Autodesk Inventor part; units mm, degrees
ref_plane "YZ Plane" through (0, 0, 0) normal (1, 0, 0) x (0, 1, 0)
ref_plane "XZ Plane" through (0, 0, 0) normal (0, 1, 0) x (-1, 0, 0)
ref_plane "XY Plane" through (0, 0, 0) normal (0, 0, 1) x (1, 0, 0)
sketch "Sketch1" plane through (0, 0, 0) normal (1, 0, 0) x (0, 1, 0)
  line L0 (-105, -75) -> (105, -75)
  line L1 (105, -75) -> (105, 75)
  line L2 (105, 75) -> (-105, 75)
  line L3 (-105, 75) -> (-105, -75)
  line L4 (-105, -75) -> (105, 75) construction
  line L5 (105, -75) -> (-105, 75) construction
  point P0 (0, 0)
  point P1 (0, 0)
  point P2 (0, 0)
  dimension "d0" = 150
  dimension "d1" = 210
extrude "Extrusion1" add sketch "Sketch1" along normal blind 6
sketch "Sketch2" plane through (6, 0, 0) normal (1, 0, 0) x (0, 0, -1)
  line L0 (75, -105) -> (75, 105)
  line L1 (-75, -105) -> (75, -105)
  line L2 (75, 105) -> (100, 105)
  line L3 (100, 105) -> (100, 80)
  line L4 (100, 80) -> (75, 30)
  line L5 (75, 30) -> (75, 105)
  line L6 (75, -105) -> (75, -5)
  line L7 (75, -5) -> (100, -55)
  line L8 (100, -55) -> (100, -105)
  line L9 (100, -105) -> (75, -105)
  point P0 (0, 0)
  dimension "d4" = 25
  dimension "d5" = 50
  dimension "d25" = 50
extrude "Extrusion2" add sketch "Sketch2" against normal blind 6
sketch "Sketch3" plane through (6, 0, 0) normal (1, 0, 0) x (0, 0, -1)
  line L0 (-75, 105) -> (-75, -105)
  line L1 (-75, -105) -> (100, -105)
  line L2 (100, -105) -> (100, -55)
  line L3 (-75, 105) -> (-25, -105)
  line L4 (-25, -105) -> (-75, -105)
  line L5 (-75, -105) -> (-75, 105)
  point P0 (0, 0)
  dimension "d8" = 50
extrude "Extrusion3" cut sketch "Sketch3" against normal through all
sketch "Sketch4" plane through (6, 0, 0) normal (1, 0, 0) x (0, 0, -1)
  line L0 (-25, -105) -> (100, -105)
  line L1 (100, -105) -> (100, -55)
  line L2 (-16.9, -105) -> (91.9, -105)
  line L3 (91.9, -105) -> (91.9, -111)
  line L4 (91.9, -111) -> (-16.9, -111)
  line L5 (-16.9, -111) -> (-16.9, -105)
  point P0 (0, 0)
  dimension "d11" = 8.1
  dimension "d12" = 8.1
  dimension "d13" = 6
extrude "Extrusion4" add sketch "Sketch4" against normal blind 6
sketch "Sketch5" plane through (6, 0, 0) normal (1, 0, 0) x (0, 0, -1)
  line L0 (-75, 105) -> (-25, -105)
  line L1 (91.9, -105) -> (100, -105)
  line L2 (100, 80) -> (100, 105)
  line L3 (100, 105) -> (-75, 105)
  circle A0 centre (-12.5, -92.5) radius 2.7
  circle A1 centre (87.5, -67.5) radius 2.7
  circle A2 centre (87.5, 92.5) radius 2.7
  circle A3 centre (-56.5476, 92.5) radius 2.7
  line L4 (-12.5, -92.5) -> (-56.5476, 92.5) construction
  line L5 (-25, -105) -> (-16.9, -105)
  point P0 (0, 0)
  dimension "d17" = 12.5
  dimension "d18" = 12.5
  dimension "d19" = 12.5
  dimension "d21" = 5.4
  dimension "d22" = 37.5
  dimension "d26" = 12.5
extrude "Extrusion5" cut sketch "Sketch5" against normal through all
fillet "Fillet1" radius 2 10 edges at (3, -111, 16.9) (3, -105, 25) (3, -111, -91.9) (3, -105, -100) (3, 105, 75) (3, 105, -100) (3, 80, -100) (3, 30, -75) (3, -5, -75) (3, -55, -100)
properties part number "BottomRightSide"
The listing builds one solid part. Answer for the finished solid, in the listing's coordinates (mm). A direction names the side the tool comes from. Coordinates: 2 decimals unless noted, no trailing zeros. Order: outer loops, then holes, each group sorted by start corner. A loop starts at its lowest first (then second) coordinate and runs counter-clockwise, first axis right, second up. Notation, with made-up numbers: (79.25, 36) -> (122.25, 36) arc R18 ccw to (122.25, 64) -> close; hole circle Ø5 at (-26.5, 70.25). An arc over 180 degrees is marked (long way). Answer in a Markdown table with one row per item. Add a question column.
Item 1: Which of the six approach directions +Z, -Z, +X, -X, +Y, -Y give full straight-line access (tool end or side, diameter ignored) to faces 1 (the face through (3.042, -95.136, 13.085)), 2 (the face through (3, -105, -95)), 3 (the face through (3, -105, 20)), 4 (the face through (3, 92, -100)), 5 (the face through (3.04, -29.66, -87.33))?
Item 2: Find section C-C (z = -87.5). Write down the section's boundary in (x, y).
Item 3: Find the intervals of material crossed by L1, parallel to Y at x = 3.2, z = 12.5; L2, parallel to Y at x = 1.5, z = -86.5; L3, parallel to Y at x = 4.55, z = -87.5, in increasing order. Write a range as from..to.
Item 4: Find section B-B (x = 3.3). Write down the section's boundary in (y, z).
Item 5: Find section D-D (y = -92.5). Write down the section's boundary in (x, z), then the cut area to 3 significant figures.
Item 6: Find section A-A (z = 12.5). Write down the section's boundary in (x, y), then the cut area to 3 significant figures.
Item 7: Each of these flat-tipped pins is pushed along its axis until it touches: P1, Ø3, axis at x = 3, y = -72, coming from the +Z side; P2, Ø3, axis at x = 2, z = -96, coming from the -Y side; P3, Ø1.8, axis at x = 4, y = 14, coming from the -Z side. Where does it stop, or does it pass through?
Item 8: Determine the mould class of faces 6 (the face through (3, -111, -38)), 7 (the face through (3, 12, -75)), 8 (the face through (3.042, -70.136, -86.915)) for opening direction Z: +Z half, -Z half, draft (parallel to the pull), parting line (faces both ways), or undercut.
Result set:
| question | item | result |
|---|---|---|
| 1 | face 1 | +X, -X |
| 1 | face 2 | -Z, +X, -X, -Y |
| 1 | face 3 | +Z, +X, -X, -Y |
| 1 | face 4 | -Z, +X, -X, +Y, -Y |
| 1 | face 5 | -Z, +X, -X |
| 2 | outline | (0, -111) -> (6, -111) -> (6, -70.2) -> (0, -70.2) -> close; (0, -64.8) -> (6, -64.8) -> (6, -30) -> (0, -30) -> close; (0, 55) -> (6, 55) -> (6, 89.8) -> (0, 89.8) -> close; (0, 95.2) -> (6, 95.2) -> (6, 105) -> (0, 105) -> close |
| 3 | L1 | y = -111..-95.2, -89.8..105 |
| 3 | L2 | y = -111..-70.01, -64.99..-28, 53..89.99, 95.01..105 |
| 3 | L3 | y = -111..-70.2, -64.8..-30, 55..89.8, 95.2..105 |
| 4 | outline | (-111, -89.9) arc R2 ccw to (-109, -91.9) -> (-105, -91.9) -> (-105, -98) arc R2 ccw to (-103, -100) -> (-55.47, -100) arc R2 ccw to (-54.58, -99.79) -> (-5.42, -75.21) arc R2 cw to (-4.53, -75) -> (29.53, -75) arc R2 cw to (30.42, -75.21) -> (79.58, -99.79) arc R2 ccw to (80.47, -100) -> (103, -100) arc R2 ccw to (105, -98) -> (105, 72.47) arc R2 ccw to (102.54, 74.41) -> (-103.46, 25.37) arc R2 ccw to (-105, 23.42) -> (-105, 16.9) -> (-109, 16.9) arc R2 ccw to (-111, 14.9) -> close; hole circle Ø5.4 at (-92.5, 12.5); hole circle Ø5.4 at (-67.5, -87.5); hole circle Ø5.4 at (92.5, -87.5); hole circle Ø5.4 at (92.5, 56.55) |
| 5 | outline | (0, -100) -> (6, -100) -> (6, 9.8) -> (0, 9.8) -> close; (0, 15.2) -> (6, 15.2) -> (6, 27.98) -> (0, 27.98) -> close |
| 5 | area | 735 mm² |
| 6 | outline | (0, -111) -> (6, -111) -> (6, -95.2) -> (0, -95.2) -> close; (0, -89.8) -> (6, -89.8) -> (6, 105) -> (0, 105) -> close |
| 6 | area | 1,260 mm² |
| 7 | P1 | stops at z = 33.21 |
| 7 | P2 | stops at y = -105 |
| 7 | P3 | stops at z = -75 |
| 8 | face 6 | draft |
| 8 | face 7 | -Z half |
| 8 | face 8 | undercut |
